from build123d import *

# Parameters (mm, degrees)
SKETCH1_W            = 140
SKETCH1_H            = 65
BOSS_EXTRUDE1_DEPTH  = 12.5
SKETCH3_W            = 130
SKETCH3_H            = 7.5
CUT_EXTRUDE1_DEPTH   = 155.858806659
FILLET1_R            = 5
SKETCH4_W            = 7.5
SKETCH4_H            = 7.5
BOSS_EXTRUDE2_DEPTH  = 4
SKETCH5_R            = 1.65
CUT_EXTRUDE2_DEPTH   = 2.5
SKETCH5_3_R          = 1.65
CUT_EXTRUDE3_DEPTH   = 154.222876882
FILLET2_R            = 8
FILLET2_OF_MIRROR1_R = 8
SKETCH7_R            = 8.4
BOSS_EXTRUDE3_DEPTH  = 11
FILLET3_R            = 1
CHAMFER1_SIZE        = 3


with BuildPart() as part:
    # Sketch1 → Boss-Extrude1 (new body)
    with BuildSketch(Plane.XY):
        with Locations((70, 32.5)):
            Rectangle(SKETCH1_W, SKETCH1_H)
    extrude(amount=BOSS_EXTRUDE1_DEPTH)

    # Sketch3 → Cut-Extrude1 (cut, through all)
    with BuildSketch(Plane(origin=(0, 65, 0), x_dir=(1, 0, 0), z_dir=(0, 1, 0))):
        with Locations((70, -8.75)):
            Rectangle(SKETCH3_W, SKETCH3_H)
    extrude(amount=-CUT_EXTRUDE1_DEPTH, mode=Mode.SUBTRACT)

    # Fillet1
    fillet1_edges = [part.edges().sort_by_distance(p)[0] for p in [
        (140, 32.5, 0),
        (0, 32.5, 0),
    ]]
    fillet(fillet1_edges, radius=FILLET1_R)

    # Sketch4 → Boss-Extrude2 (add)
    with BuildSketch(Plane.XZ):
        with Locations((8.75, 8.75)):
            Rectangle(SKETCH4_W, SKETCH4_H)
        with Locations((131.25, 8.75)):
            Rectangle(SKETCH4_W, SKETCH4_H)
    boss_extrude2 = extrude(amount=-BOSS_EXTRUDE2_DEPTH)

    # Sketch5 → Cut-Extrude2 (cut)
    # profile 1 of 2: a face of its own
    with BuildSketch(Plane(origin=(0, 4, 0), x_dir=(1, 0, 0), z_dir=(0, 1, 0))):
        Polygon((134.425426481, -8.75), (132.83771324, -6), (129.66228676, -6), (128.074573519, -8.75), (129.66228676, -11.5), (132.83771324, -11.5), align=None)
        with Locations(Location((131.25, -8.75, 0), (0, 0, 270))):
            Circle(SKETCH5_R, mode=Mode.SUBTRACT)
    # profile 2 of 2: a face of its own
    with BuildSketch(Plane(origin=(0, 4, 0), x_dir=(1, 0, 0), z_dir=(0, 1, 0))):
        Polygon((10.33771324, -6), (11.925426481, -8.75), (10.33771324, -11.5), (7.16228676, -11.5), (5.574573519, -8.75), (7.16228676, -6), align=None)
        with Locations(Location((8.75, -8.75, 0), (0, 0, 90))):
            Circle(SKETCH5_R, mode=Mode.SUBTRACT)
    cut_extrude2 = extrude(amount=-CUT_EXTRUDE2_DEPTH, mode=Mode.SUBTRACT)

    # Sketch5<3> → Cut-Extrude3 (cut, through all)
    with BuildSketch(Plane(origin=(0, 4, 0), x_dir=(1, 0, 0), z_dir=(0, 1, 0))):
        with Locations(Location((8.75, -8.75, 0), (0, 0, 270))):
            Circle(SKETCH5_3_R)
        with Locations(Location((131.25, -8.75, 0), (0, 0, 270))):
            Circle(SKETCH5_3_R)
    cut_extrude3 = extrude(amount=-CUT_EXTRUDE3_DEPTH, mode=Mode.SUBTRACT)

    # Fillet2
    # the kernel refuses this fillet: 8 mm, written as the material it adds along each edge
    with BuildSketch(Plane(origin=(127.5, 0, 5), x_dir=(-1, 0, 0), z_dir=(0, 1, 0))) as fillet2_piece_1:
        with BuildLine():
            CenterArc((7.984359711, 8), FILLET2_R, 183.583321698, 86.416678302)
            Line((0, 7.5), (-0.159687194, 7.49))
            ThreePointArc((-0.159687194, 7.49), (-0.16, 3.75), (-0.16, 0))
            Line((-0.16, 0), (0, -0.16))
            Line((0, -0.16), (7.984359711, -0.16))
            Line((7.984359711, -0.16), (7.984359711, 0))
        make_face()
    extrude(amount=4)
    with BuildSketch(Plane(origin=(12.5, 0, 5), x_dir=(1, 0, 0), z_dir=(0, 1, 0))) as fillet2_piece_2:
        with BuildLine():
            CenterArc((7.984359711, -8), FILLET2_R, 90, 86.416678302)
            Line((0, -7.5), (-0.159687194, -7.49))
            ThreePointArc((-0.159687194, -7.49), (-0.16, -3.75), (-0.16, 0))
            Line((-0.16, 0), (0, 0.16))
            Line((0, 0.16), (7.984359711, 0.16))
            Line((7.984359711, 0.16), (7.984359711, 0))
        make_face()
    extrude(amount=4)

    # Mirror1: Boss-Extrude2, Cut-Extrude2, Cut-Extrude3 across plane
    add(boss_extrude2.mirror(Plane.ZX.offset(32.5)))
    add(cut_extrude2.mirror(Plane.ZX.offset(32.5)), mode=Mode.SUBTRACT)
    add(cut_extrude3.mirror(Plane.ZX.offset(32.5)), mode=Mode.SUBTRACT)

    # Fillet2 of Mirror1
    # the kernel refuses this fillet: 8 mm, written as the material it adds along each edge
    with BuildSketch(Plane(origin=(127.5, 65, 5), x_dir=(0, 0, 1), z_dir=(0, -1, 0))) as fillet2_of_mirror1_piece_1:
        with BuildLine():
            CenterArc((8, 7.984359711), FILLET2_OF_MIRROR1_R, 180, 86.416678302)
            Line((0, 7.984359711), (-0.16, 7.984359711))
            Line((-0.16, 7.984359711), (-0.16, 0))
            Line((-0.16, 0), (0, -0.16))
            ThreePointArc((0, -0.16), (3.75, -0.16), (7.49, -0.159687194))
            Line((7.49, -0.159687194), (7.5, 0))
        make_face()
    extrude(amount=4)
    with BuildSketch(Plane(origin=(12.5, 65, 5), x_dir=(0, 0, 1), z_dir=(0, -1, 0))) as fillet2_of_mirror1_piece_2:
        with BuildLine():
            CenterArc((8, -7.984359711), FILLET2_OF_MIRROR1_R, 93.583321698, 86.416678302)
            Line((0, -7.984359711), (-0.16, -7.984359711))
            Line((-0.16, -7.984359711), (-0.16, 0))
            Line((-0.16, 0), (0, 0.16))
            ThreePointArc((0, 0.16), (3.75, 0.16), (7.49, 0.159687194))
            Line((7.49, 0.159687194), (7.5, 0))
        make_face()
    extrude(amount=4)

    # Sketch7 → Boss-Extrude3 (add)
    with BuildSketch(Plane.XY.offset(5)):
        with Locations(Location((121, 42.7, 0), (0, 0, 180))):
            Circle(SKETCH7_R)
        with Locations(Location((19, 42.7, 0), (0, 0, 180))):
            Circle(SKETCH7_R)
    extrude(amount=BOSS_EXTRUDE3_DEPTH)

    # Fillet3
    fillet3_edges = [part.edges().sort_by_distance(p)[0] for p in [
        (129.4, 42.7, 16),
        (27.4, 42.7, 16),
    ]]
    fillet(fillet3_edges, radius=FILLET3_R)

    # Chamfer1
    chamfer1_edges = [part.edges().sort_by_distance(p)[0] for p in [
        (129.4, 42.7, 5),
        (27.4, 42.7, 5),
    ]]
    chamfer(chamfer1_edges, length=CHAMFER1_SIZE)


solid = part.part
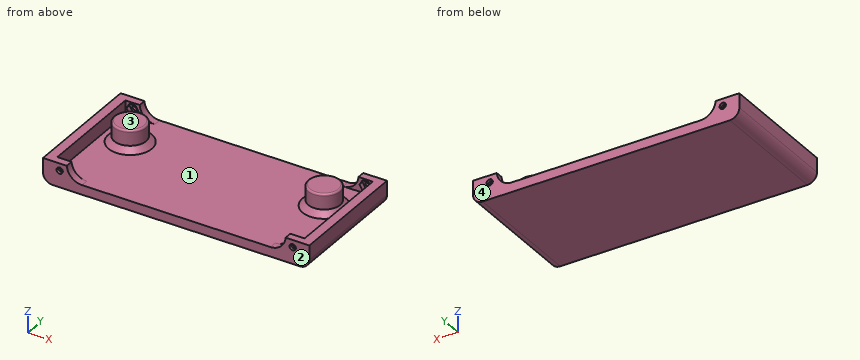
Design review of the part built by this model. Coordinates are the model's own, in mm. Face numbers are marked on the shaded views. Give positions to 0.01 mm unless a question says otherwise; leave off trailing zeros. Loops run counter-clockwise (first coordinate to the right, second up) from the corner with the lowest first, then second, coordinate; pieces in that order, holes last. Notation, with made-up numbers: M 33,20 L 56,20 A20 cw 56,52 Z; hole C -13.75,20 d1. An arc over 180 degrees is marked long. Write item = value, one per line.
Q1. We need section B-B (x = 19). Give the boundary of the cut face in (y, z).
Output values:
outline = M 0,0 L 65,0 L 65,5.14 L 61,5.14 L 61,5 L 54.1,5 L 51.1,8 L 51.1,15 A1 ccw 50.1,16 L 35.3,16 A1 ccw 34.3,15 L 34.3,8 L 31.3,5 L 4,5 L 4,5.14 L 0,5.14 Z
Q2. We need section C-C (y = 11.5). Give the boundary of the cut face in (x, z).
Output values:
outline = M 0,5 A5 ccw 5,0 L 135,0 A5 ccw 140,5 L 140,12.5 L 135,12.5 L 135,5 L 5,5 L 5,12.5 L 0,12.5 Z
Q3. To check wall thickness, follow line 1 (X direction, y = 54, z = 5.75); line 2 (X direction, y = 64.3, z = 8.75); line 3 (Z direction, x = 131.25, y = 1.2). State the ranges of each line that lie inside material, in increasing order. Write a range as [from, to].
Output values:
line_1 = [0, 5], [135, 140]
line_2 = [0, 7.1], [10.4, 13.71], [126.29, 129.6], [132.9, 140]
line_3 = [0, 7.1], [10.4, 12.5]
Q4. We need section A-A (y = 42.7). Give the boundary of the cut face in (x, z).
Output values:
outline = M 0,5 A5 ccw 5,0 L 135,0 A5 ccw 140,5 L 140,12.5 L 135,12.5 L 135,5 L 132.4,5 L 129.4,8 L 129.4,15 A1 ccw 128.4,16 L 113.6,16 A1 ccw 112.6,15 L 112.6,8 L 109.6,5 L 30.4,5 L 27.4,8 L 27.4,15 A1 ccw 26.4,16 L 11.6,16 A1 ccw 10.6,15 L 10.6,8 L 7.6,5 L 5,5 L 5,12.5 L 0,12.5 Z
Q5. We need section D-D (x = 72). Give the boundary of the cut face in (y, z).
Output values:
outline = M 0,0 L 65,0 L 65,5 L 0,5 Z
Q6. Insertion check: pin 1 (2 mm diameter, centred on x = 110, y = 33, fed in from +Z); pin 2 (8.5 mm diameter, centred on x = 16.5, z = 10.5, fed in from -Y); pin 3 (1.2 mm diameter, centred on x = 8.5, y = 62.5, fed in from +Z). Each pin has a flat end and moves straight along its axis. Give the tip position at first contact, or say it passes through.
Output values:
pin_1 = 5
pin_2 = 0
pin_3 = 12.5
Q7. Draft analysis for pull direction Y (two halves, no side actions). For the marked faces 1, 2, 3 and 4, state which applies: +Y half, -Y half, draft (parallel to the pull), parting line (faces both ways), or undercut.
Output values:
face_1 = undercut
face_2 = -Y half
face_3 = draft
face_4 = +Y half
